from build123d import *

# Parameters (mm, degrees)
SKETCH1_W           = 120
SKETCH1_H           = 40
BOSS_EXTRUDE1_DEPTH = 4
SKETCH2_R           = 1.1
SKETCH2_W           = 12.5
SKETCH2_H           = 23
CUT_EXTRUDE1_DEPTH  = 5
SKETCH3_W           = 105.5
SKETCH3_H           = 23.4
CUT_EXTRUDE2_DEPTH  = 5


with BuildPart() as part:
    # Sketch1 → Boss-Extrude1 (new body)
    with BuildSketch(Plane(origin=(0, 0, 0), x_dir=(1, 0, 0), z_dir=(0, 1, 0))):
        Rectangle(SKETCH1_W, SKETCH1_H)
    extrude(amount=BOSS_EXTRUDE1_DEPTH)

    # Sketch2 → Cut-Extrude1 (cut, through all)
    with BuildSketch(Plane(origin=(0, 4, 0), x_dir=(1, 0, 0), z_dir=(0, 1, 0))):
        with Locations((-44.998568235, 13.510712966)):
            Circle(SKETCH2_R)
        with Locations((-44.998568235, -13.5)):
            Circle(SKETCH2_R)
        with Locations((-29.998568235, 13.510712966)):
            Circle(SKETCH2_R)
        with Locations((-29.998568235, -13.5)):
            Circle(SKETCH2_R)
        with Locations((-14.998568235, 13.510712966)):
            Circle(SKETCH2_R)
        with Locations((-14.998568235, -13.5)):
            Circle(SKETCH2_R)
        with Locations((0.001431765, 13.510712966)):
            Circle(SKETCH2_R)
        with Locations((0.001431765, -13.5)):
            Circle(SKETCH2_R)
        with Locations((15.001431765, 13.510712966)):
            Circle(SKETCH2_R)
        with Locations((15.001431765, -13.5)):
            Circle(SKETCH2_R)
        with Locations((30.001431765, 13.510712966)):
            Circle(SKETCH2_R)
        with Locations((30.001431765, -13.5)):
            Circle(SKETCH2_R)
        with Locations((45.001431765, 13.510712966)):
            Circle(SKETCH2_R)
        with Locations((45.001431765, -13.5)):
            Circle(SKETCH2_R)
        with Locations((-29.998568235, 0)):
            Rectangle(SKETCH2_W, SKETCH2_H)
        with Locations((-44.998568235, 0)):
            Rectangle(SKETCH2_W, SKETCH2_H)
        with Locations((-14.998568235, 0)):
            Rectangle(SKETCH2_W, SKETCH2_H)
        with Locations((0.001431765, 0)):
            Rectangle(SKETCH2_W, SKETCH2_H)
        with Locations((15.001431765, 0)):
            Rectangle(SKETCH2_W, SKETCH2_H)
        with Locations((30.001431765, 0)):
            Rectangle(SKETCH2_W, SKETCH2_H)
        with Locations((45.001431765, 0)):
            Rectangle(SKETCH2_W, SKETCH2_H)
    extrude(amount=-CUT_EXTRUDE1_DEPTH, mode=Mode.SUBTRACT)

    # Sketch3 → Cut-Extrude2 (cut, through all)
    with BuildSketch(Plane(origin=(0, 4, 0), x_dir=(1, 0, 0), z_dir=(0, 1, 0))):
        with Locations((0.001431765, 0)):
            Rectangle(SKETCH3_W, SKETCH3_H)
    extrude(amount=-CUT_EXTRUDE2_DEPTH, mode=Mode.SUBTRACT)


solid = part.part
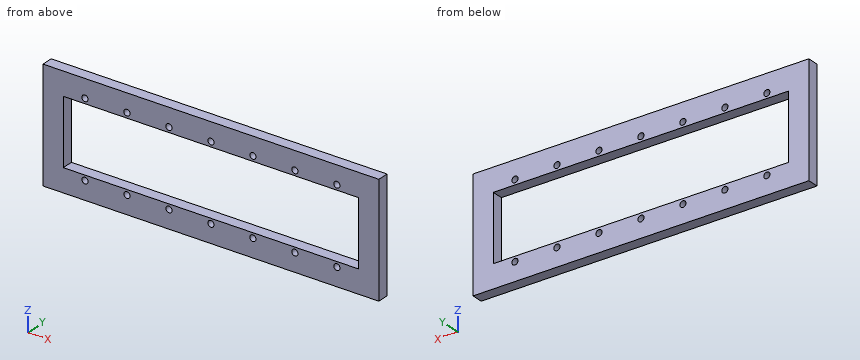
CAD build for the part. Positions are in the model's coordinates, mm. Round coordinates to 2 decimals unless told otherwise and drop trailing zeros. Loops run counter-clockwise (first coordinate to the right, second up) from the corner with the lowest first, then second, coordinate; pieces in that order, holes last. Notation, with made-up numbers: M 0.5,48 L 26.5,48 A10 cw 26.5,52 Z; hole C -31,-9.75 d5. An arc over 180 degrees is marked long. One line per question, with ' | ' between items. Start each with the question number.
Item 1: Cut at B-B, the plane x = 35.5. Write the cut outline in (y, z), plus the area to 3 significant figures.
Item 2: Wall check: line 1 (Z direction, x = 25, y = 2.1); line 2 (X direction, y = 1.8, z = -6); line 3 (Z direction, x = 30, y = 0.4). Give the ranges that are in metal, low to high.
Item 3: Pin check, flat tips, straight feed: pin 1 Ø2.5 at (x, z) = (0, 13.5) entering from +Y; pin 2 Ø1.8 at (x, z) = (-45, -13.51) entering from -Y. Stop position of each tip, or through.
Item 4: Cut at C-C, the plane z = -4.5. Write the cut outline in (x, y), plus the area to 3 significant figures.
Item 5: Cut at A-A, the plane z = 13.5. State how many separate pieces and enclosed holes the cut face has, plus the area to 3 significant figures.
Responses:
1) outline: M 0,-20 L 4,-20 L 4,-11.7 L 0,-11.7 Z; M 0,11.7 L 4,11.7 L 4,20 L 0,20 Z | area: 66.4 mm²
2) line 1: z = -20 to -11.7, 11.7 to 20 | line 2: x = -60 to -52.75, 52.75 to 60 | line 3: z = -20 to -14.61, -12.41 to -11.7, 11.7 to 12.4, 14.6 to 20
3) pin 1: stops at y = 4 | pin 2: passes through
4) outline: M -60,0 L -52.75,0 L -52.75,4 L -60,4 Z; M 52.75,0 L 60,0 L 60,4 L 52.75,4 Z | area: 58.0 mm²
5) separate pieces: 8 | enclosed holes: 0 | area: 418 mm²
